Input: part model. Units: mm. Frame: model coordinates. A direction names the side the tool comes from. Round coordinates to 2 decimals unless told otherwise and drop trailing zeros. Loops run counter-clockwise (first coordinate to the right, second up) from the corner with the lowest first, then second, coordinate; pieces in that order, holes last. Notation, with made-up numbers: M -5.75,-14 L 1.25,-14 A23 cw 1.25,21 Z; hole C 28,63 d9. An arc over 180 degrees is marked long. Put each result on its own line as item: value. Start each with the question number.
1) Section A-A on x = -2620.5. Output: boundary loops of the cut face in (y, z), plus the area to 3 significant figures.
2) Line query: probe 1 along Y at (x, z) = (-3091.5, 5219); probe 2 along Y at (x, z) = (-2301, 5451.5); probe 3 along Y at (x, z) = (-2309, 5716). Output: solid intervals per line, ascending.
3) Section C-C on z = 6059. Output: boundary loops of the cut face in (x, y), plus the area to 3 significant figures.
4) Section D-D on x = -3036. Output: boundary loops of the cut face in (y, z), plus the area to 3 significant figures.
5) Section B-B on y = 1771.5. Output: boundary loops of the cut face in (x, z).
6) Pin query (flat end, axial travel): pin 1 (12 mm diameter, centred on x = -2101, y = 1570.5, fed in from +Z); pin 2 (3 mm diameter, centred on y = -203.5, z = 5612, fed in from -X); pin 3 (8 mm diameter, centred on x = -2665, y = 1253.5, fed in from +Z). Return the tip coordinate at first contact, or that it passes through.
7) Reachability of faces 1 (the face through (-2266, -165, 5553)), 2 (the face through (-2252.518, -181.269, 5521.596)) from +Z, -Z, +X, -X, +Y, -Y: full face, straight path, thin tool, end or side. Return the list, or none.
8) Draft query along Y for faces 3 (the face through (-2587, 2035, 5482)), 4 (the face through (-2881.635, -114.3, 5665.36)), 5 (the face through (-3134.17, 999.7, 5045.69)). Return one class per face: +Y half, -Y half, draft (parallel to the pull), parting line (faces both ways), or undercut.
from build123d import *

# Parameters (mm, degrees)
SKETCH013_R   = 701.420325
PAD013_DEPTH  = 2100
SKETCH014_R   = 315.090162
PAD014_DEPTH  = 100
SKETCH016_R   = 338.402277
PAD016_DEPTH  = 33
SKETCH027_W   = 30.567139
SKETCH027_H   = 255.999512
SKETCH027_W_2 = 34.387939
SKETCH027_H_2 = 290.387695
PAD021_DEPTH  = 10


with BuildPart() as part:
    # Sketch013 → Pad013 (new body)
    with BuildSketch(Plane.XZ):
        with Locations((-2577.543945, 5472.492188)):
            Circle(SKETCH013_R)
    extrude(amount=PAD013_DEPTH)

    # Sketch014 (on Face3 of Pad013) → Pad014 (join)
    with BuildSketch(Plane.XZ.offset(2100)):
        with Locations((-2566.849609, 5651.506348)):
            Circle(SKETCH014_R)
    extrude(amount=PAD014_DEPTH)

    # Sketch016 (on Face5 of Pad014) → Pad016 (join)
    with BuildSketch(Plane.XZ.offset(2200)):
        with Locations((-2565.115723, 5651.206055)):
            Circle(SKETCH016_R)
    extrude(amount=PAD016_DEPTH)

    # Sketch027 (on Face3 of Pad016) → Pad021 (join)
    with BuildSketch(Plane.XZ.offset(2233)):
        with Locations((-2775.766723, 5650.032471)):
            Rectangle(SKETCH027_W, SKETCH027_H)
        with Locations((-2368.842407, 5667.226562)):
            Rectangle(SKETCH027_W_2, SKETCH027_H_2)
    extrude(amount=PAD021_DEPTH)


with BuildPart() as part_1:
    # Body013 placement: moved
    add(part.part.moved(Location((0, 2035, 0))))


solid = part_1.part
Geometry results:
1. outline: M -198,5317.37 L -165,5317.37 L -165,5341.02 L -65,5341.02 L -65,4772.39 L 2035,4772.39 L 2035,6172.6 L -65,6172.6 L -65,5962 L -165,5962 L -165,5985.05 L -198,5985.05 Z
1. area: 3,020,000 mm²
2. probe 1: y = -65 to 2035
2. probe 2: y = -198 to -165, -65 to 2035
2. probe 3: y = -198 to 2035
3. outline: M -2962.25,-65 L -2192.84,-65 L -2192.84,2035 L -2962.25,2035 Z
3. area: 1,620,000 mm²
4. outline: M -65,4941.64 L 2035,4941.64 L 2035,6003.35 L -65,6003.35 Z
4. area: 2,230,000 mm²
5. outline: C -2577.54,5472.49 d1402.84
6. pin 1: stops at z = 5992.66
6. pin 2: stops at x = -2791.05
6. pin 3: stops at z = 6168.93
7. face 1: none
7. face 2: -Y
8. face 3: +Y half
8. face 4: undercut
8. face 5: draft
